Here's how the part is built. I have some questions about the finished solid (model axes, mm). Coordinates: 2 decimals unless noted, no trailing zeros. Write each loop counter-clockwise with the first axis right and the second up, starting at its lowest first coordinate (ties: lowest second). Pieces come first, ordered by that corner, then holes.
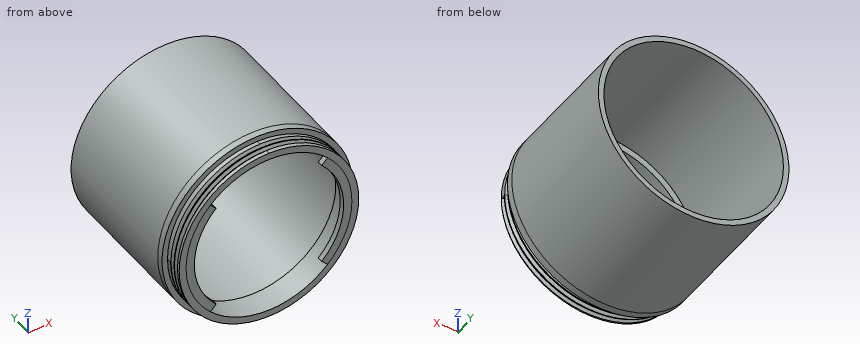
```python
from build123d import *
from build123d.topology import SkipClean

# Parameters (mm, degrees)
SKETCH1_R           = 32.75
SKETCH1_R_2         = 30.25
BOSS_EXTRUDE1_DEPTH = 6.75
SKETCH2_R           = 34.75
SKETCH2_R_2         = 30.25
BOSS_EXTRUDE2_DEPTH = 2.5
THREAD1_PITCH       = 2
BOSS_EXTRUDE3_DEPTH = 2
SKETCH5_R           = 34.75
SKETCH5_R_2         = 32.75
BOSS_EXTRUDE4_DEPTH = 50


with BuildPart() as part:
    # Sketch1 → Boss-Extrude1 (new body)
    with BuildSketch(Plane(origin=(0, 0, 0), x_dir=(1, 0, 0), z_dir=(0, 1, 0))):
        with Locations(Location((0, 0, 0), (0, 0, 270))):
            Circle(SKETCH1_R)
        with Locations(Location((0, 0, 0), (0, 0, 270))):
            Circle(SKETCH1_R_2, mode=Mode.SUBTRACT)
    extrude(amount=BOSS_EXTRUDE1_DEPTH)

    # Sketch2 → Boss-Extrude2 (add)
    with BuildSketch(Plane(origin=(0, 6.75, 0), x_dir=(1, 0, 0), z_dir=(0, 1, 0))):
        with Locations(Location((0, 0, 0), (0, 0, 270))):
            Circle(SKETCH2_R)
        with Locations(Location((0, 0, 0), (0, 0, 270))):
            Circle(SKETCH2_R_2, mode=Mode.SUBTRACT)
    extrude(amount=BOSS_EXTRUDE2_DEPTH)

    # Thread1: the profile of Thread Profile1 profile screwed along a right-hand helix of 2.5 turns, 10 arcs to a turn; built about Z, then put on its axis
    with SkipClean():  # the faces are left unmerged after this step: merging them gives an invalid solid
        thread1_z = Axis((0, 0, 0), (0, 0, 1))
        thread1_corners = [(32.7503, 0, -0.000173205), (32.7503, 0, 1.7501732), (31.66746825, 0, 1.124999997), (31.66746825, 0, 0.624999997)]
        with BuildLine(mode=Mode.PRIVATE) as thread1_profile:
            Line(thread1_corners[0], thread1_corners[1])
            Line(thread1_corners[1], thread1_corners[2])
            Line(thread1_corners[2], thread1_corners[3])
            Line(thread1_corners[3], thread1_corners[0])
        thread1_cap = Face(thread1_profile.wire())
        thread1_turn_angles = [0, 18, 36, 54, 72, 90, 108, 126, 144, 162, 180, 198, 216, 234, 252, 270, 288, 306, 324, 342, 360]
        thread1_turn_weights = [1, 0.9510565162951535, 1, 0.9510565162951535, 1, 0.9510565162951535, 1, 0.9510565162951535, 1, 0.9510565162951535, 1, 0.9510565162951535, 1, 0.9510565162951535, 1, 0.9510565162951535, 1, 0.9510565162951535, 1, 0.9510565162951535, 1]
        thread1_turn_rails = [Edge.make_bspline([Vector(p[0], p[1], 0).rotate(thread1_z, thread1_turn_angles[k]) / thread1_turn_weights[k] + Vector(0, 0, p[2] + THREAD1_PITCH * thread1_turn_angles[k] / 360) for k in range(21)], [0, 0, 0, 1, 1, 2, 2, 3, 3, 4, 4, 5, 5, 6, 6, 7, 7, 8, 8, 9, 9, 10, 10, 10], 2, thread1_turn_weights) for p in thread1_corners]
        thread1_turn_sides = [Face.make_surface_from_curves(thread1_turn_rails[p[0]], thread1_turn_rails[p[1]]) for p in [(0, 1), (1, 2), (2, 3), (3, 0)]]
        thread1_last_angles = [720, 738, 756, 774, 792, 810, 828, 846, 864, 882, 900]
        thread1_last_weights = [1, 0.9510565162951535, 1, 0.9510565162951535, 1, 0.9510565162951535, 1, 0.9510565162951535, 1, 0.9510565162951535, 1]
        thread1_last_rails = [Edge.make_bspline([Vector(p[0], p[1], 0).rotate(thread1_z, thread1_last_angles[k]) / thread1_last_weights[k] + Vector(0, 0, p[2] + THREAD1_PITCH * thread1_last_angles[k] / 360) for k in range(11)], [0, 0, 0, 1, 1, 2, 2, 3, 3, 4, 4, 5, 5, 5], 2, thread1_last_weights) for p in thread1_corners]
        thread1_last_sides = [Face.make_surface_from_curves(thread1_last_rails[p[0]], thread1_last_rails[p[1]]) for p in [(0, 1), (1, 2), (2, 3), (3, 0)]]
        thread1 = Plane(origin=(0, 0, 0), x_dir=(1, 0, 0), z_dir=(0, 1, 0)) * Solid(Shell([*[p.moved(Location((0, 0, THREAD1_PITCH * i))) for i in range(2) for p in thread1_turn_sides], *thread1_last_sides, thread1_cap, thread1_cap.rotate(thread1_z, 900).moved(Location((0, 0, THREAD1_PITCH * 900 / 360)))]))
        add(thread1, mode=Mode.SUBTRACT)

    # Sketch3 → Boss-Extrude3 (add)
    with SkipClean():  # the faces are left unmerged after this step: merging them gives an invalid solid
        with BuildSketch(Plane.XZ):
            with BuildLine():
                Line((19.268659787, 19.268659787), (21.389980131, 21.389980131))
                ThreePointArc((21.389980131, 21.389980131), (30.25, 0), (21.389980131, -21.389980131))
                Line((21.389980131, -21.389980131), (19.268659787, -19.268659787))
                ThreePointArc((19.268659787, -19.268659787), (27.25, 0), (19.268659787, 19.268659787))
            make_face()
            with BuildLine():
                Line((-19.268659787, 19.268659787), (-21.389980131, 21.389980131))
                ThreePointArc((-21.389980131, 21.389980131), (-30.25, 0), (-21.389980131, -21.389980131))
                Line((-21.389980131, -21.389980131), (-19.268659787, -19.268659787))
                ThreePointArc((-19.268659787, -19.268659787), (-27.25, 0), (-19.268659787, 19.268659787))
            make_face()
        extrude(amount=-BOSS_EXTRUDE3_DEPTH)

    # Sketch5 → Boss-Extrude4 (add)
    with SkipClean():  # the faces are left unmerged after this step: merging them gives an invalid solid
        with BuildSketch(Plane(origin=(0, 9.25, 0), x_dir=(1, 0, 0), z_dir=(0, 1, 0))):
            with Locations(Location((0, 0, 0), (0, 0, 270))):
                Circle(SKETCH5_R)
            with Locations(Location((0, 0, 0), (0, 0, 270))):
                Circle(SKETCH5_R_2, mode=Mode.SUBTRACT)
        extrude(amount=BOSS_EXTRUDE4_DEPTH)


solid = part.part
```
1) Imagine slicing it at A-A on y = 53.5. Please give me the cut outline in (x, z), then the cut area to 3 significant figures.
Values follow:
outline: circle Ø69.5 at (0, 0); hole circle Ø65.5 at (0, 0)
area: 424 mm2
2) Will these pins go through, and if not, where does the flat tip stop? pin 1 (12 mm diameter, centred on x = 17.5, y = 31.5, fed in from +Z); pin 2 (12 mm diameter, centred on y = 25, z = -14.5, fed in from +X); pin 3 (5 mm diameter, centred on x = -4, z = -27.5, fed in from +Y); pin 4 (12 mm diameter, centred on x = -19.5, z = 23.5, fed in from +Y).
Values follow:
pin 1: stops at z = 32.79
pin 2: stops at x = 33.69
pin 3: stops at y = 9.25
pin 4: stops at y = 59.25
3) I need wall thicknesses on probe 1 along X at (y, z) = (7, 0); probe 2 along Y at (x, z) = (31, -2); probe 3 along X at (y, z) = (24, 0). Which ranges of each line are inside material? Lowest first, please.
Values follow:
probe 1: x = -34.75 to -30.25, 30.25 to 34.75
probe 2: y = 0 to 9.25
probe 3: x = -34.75 to -32.75, 32.75 to 34.75
